```python
from build123d import *

# Parameters (mm, degrees)
F0_W     = 12
F0_H     = 11
F0_W_2   = 11
F0_H_2   = 10
F1_DEPTH = 28
F2_W     = 10
F2_H     = 11
F3_DEPTH = 2
F4_W     = 10
F4_H     = 11
F5_DEPTH = 2


with BuildPart() as f1:
    # F0 (on Top) → F1 (new body)
    with BuildSketch(Plane.XY):
        with Locations((-1.675564, -2.512802)):
            Rectangle(F0_W, F0_H)
        with Locations((-1.675564, -2.512802)):
            Rectangle(F0_W_2, F0_H_2, mode=Mode.SUBTRACT)
    extrude(amount=F1_DEPTH)

    # F2 (on face) → F3 (cut)
    with BuildSketch(Plane.YZ.offset(4.324436)):
        with Locations((-2.512802, 5.5)):
            Rectangle(F2_W, F2_H)
    extrude(amount=-F3_DEPTH, mode=Mode.SUBTRACT)

    # F4 (on face) → F5 (cut)
    with BuildSketch(Plane(origin=(-7.675564, 0, 0), x_dir=(0, -1, 0), z_dir=(-1, 0, 0))):
        with Locations((2.512802, 22)):
            Rectangle(F4_W, F4_H)
    extrude(amount=-F5_DEPTH, mode=Mode.SUBTRACT)


solid = f1.part
```
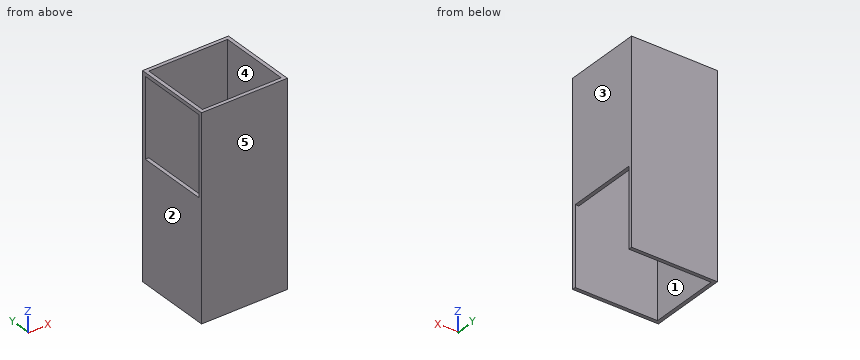
Can you work these out from the model? Positions are in its coordinate system, mm. Face numbers are marked on the shaded views. A direction names the side the tool comes from. Coordinates: 2 decimals unless noted, no trailing zeros. Loops run counter-clockwise (first coordinate to the right, second up) from the corner with the lowest first, then second, coordinate; pieces in that order, holes last.
1) Which directions (+Z, -Z, +X, -X, +Y, -Y) give clear straight access to the entire face, cutting with the end or side of a thin tool? Please do the marked faces 1 and 2.
2) Imagine slicing it at D-D on z = 4.5. List the corners of the cut face in (x, y) for me.
3) I need wall thicknesses on probe 1 along Y at (x, z) = (0.75, 23); probe 2 along X at (y, z) = (-3.5, 26.75); probe 3 along X at (y, z) = (1.5, 15). Which ranges of each line are inside material? Lowest first, please.
4) Thinking about a two-plate mould opening in X: for the marked faces 3, 4 and 5, which applies, pulls with the +X half, pulls with the -X half, needs draft (parallel to the pull), parting line crosses it, or undercut?
5) Imagine slicing it at B-B on z = 12.25. List the corners of the cut face in (x, y) for me.
6) For pin 1 (3 mm diameter, centred on y = -1.5, z = 5.5, fed in from +X); pin 2 (3 mm diameter, centred on x = -4.5, y = -5, fed in from +Z), each with a flat end and sliding along its axis, tell me the tip position at first contact or that it passes through.
7) Imagine slicing it at C-C on y = -2.25. List the corners of the cut face in (x, z) for me, plus the area to 3 significant figures.
8) Imagine slicing it at A-A on x = -2.25. List the corners of the cut face in (y, z) for me, plus the area to 3 significant figures.
Completed:
1. face 1: +Z, -Z
1. face 2: +Z, -Z, -X, +Y, -Y
2. outline: (-7.68, -8.01) - (4.32, -8.01) - (4.32, -7.51) - (-7.18, -7.51) - (-7.18, 2.49) - (4.32, 2.49) - (4.32, 2.99) - (-7.68, 2.99) - close
3. probe 1: y = -8.01 to -7.51, 2.49 to 2.99
3. probe 2: x = 3.82 to 4.32
3. probe 3: x = -7.68 to -7.18, 3.82 to 4.32
4. face 3: pulls with the +X half
4. face 4: undercut
4. face 5: needs draft
5. outline: (-7.68, -8.01) - (4.32, -8.01) - (4.32, 2.99) - (-7.68, 2.99) - close; hole (-7.18, -7.51) - (3.82, -7.51) - (3.82, 2.49) - (-7.18, 2.49) - close
6. pin 1: stops at x = -7.18
6. pin 2: passes through
7. outline: (-7.68, 0) - (-7.18, 0) - (-7.18, 16.5) - (-7.68, 16.5) - close; (-7.68, 27.5) - (-7.18, 27.5) - (-7.18, 28) - (-7.68, 28) - close; (3.82, 11) - (4.32, 11) - (4.32, 28) - (3.82, 28) - close
7. area: 17.0 mm2
8. outline: (-8.01, 0) - (-7.51, 0) - (-7.51, 28) - (-8.01, 28) - close; (2.49, 0) - (2.99, 0) - (2.99, 28) - (2.49, 28) - close
8. area: 28.0 mm2
